Drawing for the job (mm, zero at the part's lowest x, y, z). Give positions to 0.01 mm unless a question says otherwise; leave off trailing zeros. Order: outer loops, then holes, each group sorted by start corner. A loop starts at its lowest first (then second) coordinate and runs counter-clockwise, first axis right, second up. Notation, with made-up numbers: M 9,-16.5 L 66,-16.5 A31 cw 66,14.5 Z; hole C -7.75,29.5 d4. An arc over 180 degrees is marked long. One line per item, written item: value.
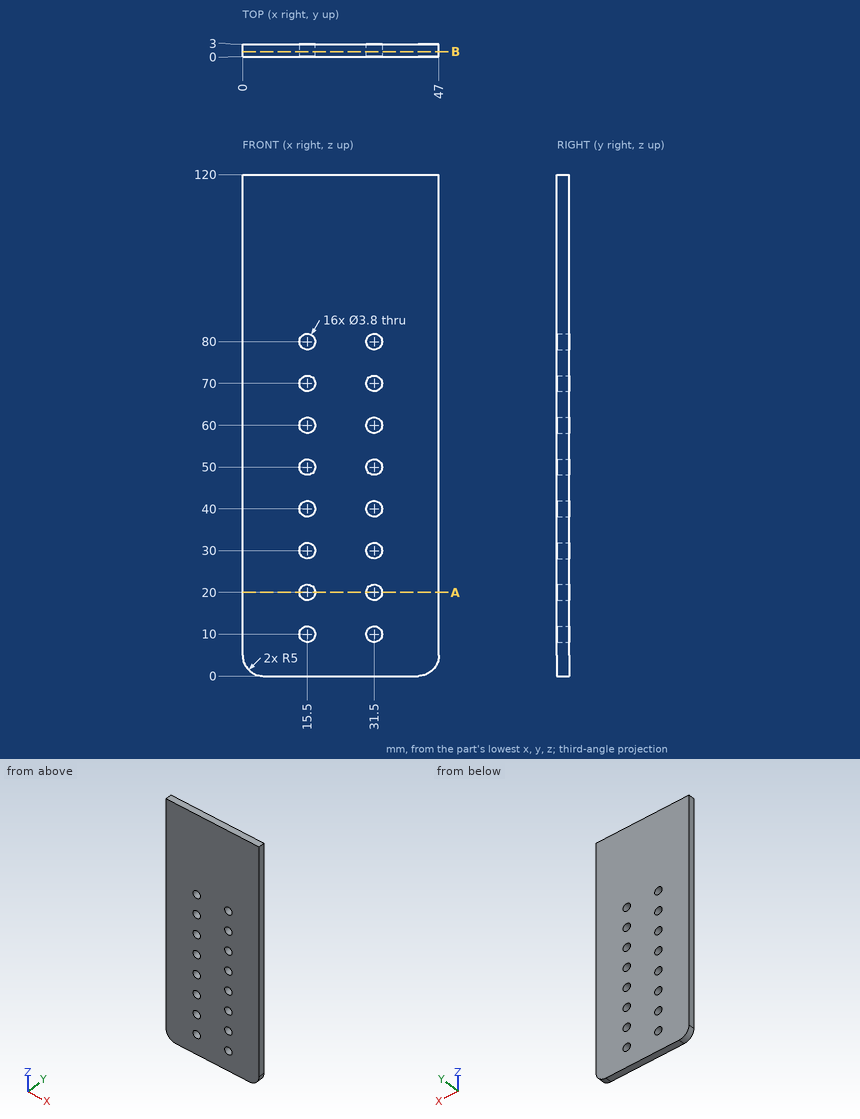
1) Saw through at A-A, the plane z = 20. Write the cut outline in (x, y), then the cut area to 3 significant figures.
Check values:
outline: M 0,0 L 13.6,0 L 13.6,3 L 0,3 Z; M 17.4,0 L 29.6,0 L 29.6,3 L 17.4,3 Z; M 33.4,0 L 47,0 L 47,3 L 33.4,3 Z
area: 118 mm^2
2) Drill centre lines: probe 1 along X at (y, z) = (1.1, 70); probe 2 along X at (y, z) = (2.35, 61.5); probe 3 along Z at (x, y) = (4.5, 1.2). Where is each one in solid material? Low to high. Write a range as from..to.
Check values:
probe 1: 0..13.6, 17.4..29.6, 33.4..47
probe 2: 0..14.33, 16.67..30.33, 32.67..47
probe 3: 0.03..120
3) Saw through at B-B, the plane y = 1.2. Give the number of separate pieces and of enclosed holes in the cut face, then the cut area to 3 significant figures.
Check values:
separate pieces: 1
enclosed holes: 16
area: 5,450 mm^2
4) Pin check, flat tips, straight feed: pin 1 (3.5 mm diameter, centred on x = 15.5, z = 50, fed in from -Y); pin 2 (5 mm diameter, centred on x = 31.5, z = 40, fed in from +Y). Stop position of each tip, or through.
Check values:
pin 1: through
pin 2: y = 3
